For this review, take the finished solid that the model builds, in its own axes (mm). Round coordinates to 2 decimals unless told otherwise and drop trailing zeros. Loops run counter-clockwise (first coordinate to the right, second up) from the corner with the lowest first, then second, coordinate; pieces in that order, holes last.
1. Consider section C-C on z = -3.5. State the section outline as (x, y) points, then the cut area to 3 significant figures.
2. To check wall thickness, follow line 1 along Z through (x, y) = (1, 0.15); line 2 along X through (y, z) = (0.7, -8.5); line 3 along Z through (x, y) = (12, 0.25). State the ranges of each line that lie inside material, in increasing order.
3. Consider section A-A on x = 10.5. State the section outline as (y, z) points, then the cut area to 3 significant figures.
4. Consider section D-D on z = 10. State the section outline as (x, y) points, then the cut area to 3 significant figures.
5. Consider section B-B on y = 0.2. State the section outline as (x, z) points.
from build123d import *

# Parameters (mm, degrees)
SKETCH_1_W          = 27
SKETCH_1_H          = 38
EXTRUDE_1_DEPTH     = 0.8
FILLET_1_R          = 1.2
CUT_EXTRUDE_1_REACH = 2.8
SKETCH_2_W          = 5
SKETCH_2_H          = 9.5
SKETCH_3_W          = 5
SKETCH_3_H          = 1
SKETCH_3_W_2        = 1
SKETCH_3_H_2        = 5
CUT_EXTRUDE_2_DEPTH = 10


with BuildPart() as part:
    # 草图1 → 凸台-拉伸1 (new body)
    with BuildSketch(Plane(origin=(0, 0, 0), x_dir=(1, 0, 0), z_dir=(0, 1, 0))):
        Rectangle(SKETCH_1_W, SKETCH_1_H)
    extrude(amount=EXTRUDE_1_DEPTH)

    # 圆角1
    fillet_1_edges = [part.edges().sort_by_distance(p)[0] for p in [
        (13.5, 0.4, 19),
        (-13.5, 0.4, 19),
        (-13.5, 0.4, -19),
        (13.5, 0.4, -19),
    ]]
    fillet(fillet_1_edges, radius=FILLET_1_R)

    # 草图2 → 切除-拉伸1 (cut, up to next)
    with BuildSketch(Plane(origin=(0, 0.8, 0), x_dir=(1, 0, 0), z_dir=(0, 1, 0)), mode=Mode.PRIVATE) as cut_extrude_1_sk1:
        with Locations((11, 5.88)):
            Rectangle(SKETCH_2_W, SKETCH_2_H)
    cut_extrude_1_tool1 = extrude(cut_extrude_1_sk1.sketch, amount=-CUT_EXTRUDE_1_REACH, mode=Mode.PRIVATE) & part.part
    add(cut_extrude_1_tool1.solids().sort_by_distance((11, 0.8, -5.88))[0], mode=Mode.SUBTRACT)

    # 草图3 → 切除-拉伸2 (cut)
    with BuildSketch(Plane(origin=(0, 0.8, 0), x_dir=(1, 0, 0), z_dir=(0, 1, 0))):
        with Locations((0, 18.5)):
            Rectangle(SKETCH_3_W, SKETCH_3_H)
        with Locations((-13, -11.5)):
            Rectangle(SKETCH_3_W_2, SKETCH_3_H_2)
        with Locations((13, -11.5)):
            Rectangle(SKETCH_3_W_2, SKETCH_3_H_2)
    extrude(amount=-CUT_EXTRUDE_2_DEPTH, mode=Mode.SUBTRACT)


solid = part.part
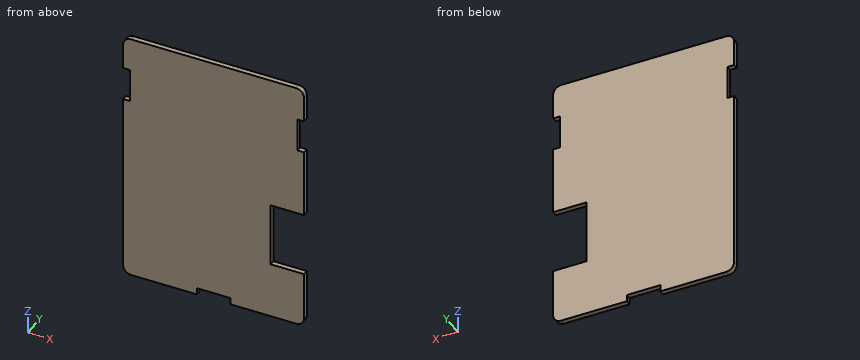
Resolved:
1. outline: (-13.5, 0) - (8.5, 0) - (8.5, 0.8) - (-13.5, 0.8) - close
1. area: 17.6 mm2
2. line 1: z = -18 to 19
2. line 2: x = -13.5 to 8.5
2. line 3: z = -19 to -10.63, -1.13 to 19
3. outline: (0, -19) - (0.8, -19) - (0.8, -10.63) - (0, -10.63) - close; (0, -1.13) - (0.8, -1.13) - (0.8, 19) - (0, 19) - close
3. area: 22.8 mm2
4. outline: (-12.5, 0) - (12.5, 0) - (12.5, 0.8) - (-12.5, 0.8) - close
4. area: 20.0 mm2
5. outline: (-13.5, -17.8) arc R1.2 ccw to (-12.3, -19) - (-2.5, -19) - (-2.5, -18) - (2.5, -18) - (2.5, -19) - (12.3, -19) arc R1.2 ccw to (13.5, -17.8) - (13.5, -10.63) - (8.5, -10.63) - (8.5, -1.13) - (13.5, -1.13) - (13.5, 9) - (12.5, 9) - (12.5, 14) - (13.5, 14) - (13.5, 17.8) arc R1.2 ccw to (12.3, 19) - (-12.3, 19) arc R1.2 ccw to (-13.5, 17.8) - (-13.5, 14) - (-12.5, 14) - (-12.5, 9) - (-13.5, 9) - close
